For this review, take the finished solid that the model builds, in its own axes (mm). Round coordinates to 2 decimals unless told otherwise and drop trailing zeros. Loops run counter-clockwise (first coordinate to the right, second up) from the corner with the lowest first, then second, coordinate; pieces in that order, holes last. Notation, with made-up numbers: M 3,-37 L 35,-37 A20 cw 35,-13 Z; hole C -28.75,88.5 d5. An arc over 180 degrees is marked long. Write item = value, one per line. Start each with the question number.
```python
from build123d import *

# Parameters (mm, degrees)
SKETCH1_W                                = 50.8
SKETCH1_H                                = 38.1
BOSS_EXTRUDE1_DEPTH                      = 25.4
CUT_SWEEP1_PROFILE_R                     = 9.525
M6_CLEARANCE_HOLE1_D                     = 6.6
M6_CLEARANCE_HOLE1_CSINK_D               = 6.65
M6_CLEARANCE_HOLE1_CSINK_ANGLE           = 90
M6_CLEARANCE_HOLE1_ON_FACE_2_D           = 6.6
M6_CLEARANCE_HOLE1_ON_FACE_2_CSINK_D     = 6.65
M6_CLEARANCE_HOLE1_ON_FACE_2_CSINK_ANGLE = 90


with BuildPart() as part:
    # Sketch1 → Boss-Extrude1 (new body)
    with BuildSketch(Plane.XY):
        Polygon((5.399653784, 95.801105715), (25.4, 19.05), (-25.4, 19.05), (-5.399653784, 95.801105715), align=None)
        Rectangle(SKETCH1_W, SKETCH1_H)
    extrude(amount=BOSS_EXTRUDE1_DEPTH)

    # Cut-Sweep1: sweep along a path in Sketch2
    with BuildLine(Plane.XY.offset(25.4)) as cut_sweep1_path:
        Line((-25.4, 0), (25.4, 0))
    # Cut-Sweep1 profile (on start of the path) → Cut-Sweep1 (sweep, cut)
    with BuildSketch(Plane(origin=(-25.4, 0, 25.4), x_dir=(0, 1, 0), z_dir=(1, 0, 0))):
        Circle(CUT_SWEEP1_PROFILE_R)
    sweep(path=cut_sweep1_path.line, mode=Mode.SUBTRACT)

    # M6 Clearance Hole1 (through all)
    with Locations(Plane(origin=(0, 0, 15.875), x_dir=(0, 1, 0), z_dir=(0, 0, 1))):
        with Locations((0, 0), (0, 15.875), (0, -15.875)):
            CounterSinkHole(M6_CLEARANCE_HOLE1_D / 2, M6_CLEARANCE_HOLE1_CSINK_D / 2, counter_sink_angle=M6_CLEARANCE_HOLE1_CSINK_ANGLE)

    # M6 Clearance Hole1 on face 2 (through all)
    with Locations(Plane(origin=(0, 89.092444953, 25.4), x_dir=(1, 0, 0), z_dir=(0, 0, 1))):
        with Locations((0, 0)):
            CounterSinkHole(M6_CLEARANCE_HOLE1_ON_FACE_2_D / 2, M6_CLEARANCE_HOLE1_ON_FACE_2_CSINK_D / 2, counter_sink_angle=M6_CLEARANCE_HOLE1_ON_FACE_2_CSINK_ANGLE)


solid = part.part
```
(1) Add section A-A on x = 0. Write out the cut boundary in (y, z) (3 decimals), and give its area (3 significant figures).
(2) Wall thickness on L1, parallel to X at y = 0, z = 5.25 (3 decimals); L2, parallel to Y at x = 1, z = 17.25; L3, parallel to Y at x = 0, z = 19.75: over which ranges is each line inside the solid? List them lowest first.
(3) For pin 1 Ø1.5 at (y, z) = (60, 22) entering from +X; pin 2 Ø6 at (y, z) = (46, 7) entering from +X; pin 3 Ø2 at (y, z) = (62.5, 3.5) entering from +X, all flat-tipped, find the tip position at first contact; note any pin that passes through.
(4) Add section B-B on z = 10.25. Write out the cut boundary in (x, y) (3 decimals), and give its area (3 significant figures).
(5) Draft analysis for pull direction X (two halves, no side actions). For faces 1 (the flat face through (0, -14, 25.4)), 2 (the cylindrical face through (-1.774, 91.875, 12.51)), 3 (the flat face through (15.26, 57.96, 12.52)), state which applies: +X half, -X half, draft (parallel to the pull), parting line (faces both ways), or undercut.
(6) Add section C-C on y = 2. Count the separate pieces of the cut face and the enclosed holes in it, and give its area (3 significant figures).
(7) Add section D-D on x = -20.5. Write out the cut boundary in (y, z) (3 decimals).
Answer sheet:
q1.outline = M -19.05,0 L -3.3,0 L -3.3,15.85 L -3.325,15.875 L -3.325,16.474 A9.525 cw -9.525,25.4 L -19.05,25.4 Z; M 3.3,0 L 85.792,0 L 85.792,25.375 L 85.767,25.4 L 9.525,25.4 A9.525 cw 3.325,16.474 L 3.325,15.875 L 3.3,15.85 Z; M 92.392,0 L 95.801,0 L 95.801,25.4 L 92.417,25.4 L 92.392,25.375 Z
q1.area = 2,500 mm²
q2.L1 = -25.4 to -19.175, -12.575 to -3.3, 3.3 to 12.575, 19.175 to 25.4
q2.L2 = -19.05 to -4.93, 4.93 to 85.95, 92.24 to 95.8
q2.L3 = -19.05 to -7.67, 7.67 to 85.79, 92.39 to 95.8
q3.pin_1 = 14.92
q3.pin_2 = 19.16
q3.pin_3 = 14.34
q4.outline = M -25.4,-19.05 L 25.4,-19.05 L 25.4,19.05 L 5.4,95.801 L -5.4,95.801 L -25.4,19.05 Z; hole C -15.875,0 d6.6; hole C 0,0 d6.6; hole C 0,89.092 d6.6; hole C 15.875,0 d6.6
q4.area = 4,160 mm²
q5.face_1 = draft
q5.face_2 = undercut
q5.face_3 = +X half
q6.separate_pieces = 4
q6.enclosed_holes = 0
q6.area = 564 mm²
q7.outline = M -19.05,0 L 37.854,0 L 37.854,25.4 L 9.525,25.4 A9.525 cw -9.525,25.4 L -19.05,25.4 Z
